Source: CAD feature listing. Evaluate the final solid. Frame: model axes, mm. A direction names the side the tool comes from. Coordinates: 2 decimals unless noted, no trailing zeros. Write each loop counter-clockwise with the first axis right and the second up, starting at its lowest first coordinate (ties: lowest second). Pieces come first, ordered by that corner, then holes. Notation, with made-up numbers: M 84.5,57.25 L 107.5,57.25 A24 cw 107.5,94.25 Z; hole C -16.5,-10.5 d6. An arc over 180 degrees is marked long. Answer as CSV lines item,"result". Start each with the question number.
1. Section C-C on z = 0.6. Return the cut outline in (x, y), plus the area to 3 significant figures.
2. Section A-A on x = 7.5. Return the cut outline in (y, z), plus the area to 3 significant figures.
3. Section B-B on y = 32. Return the cut outline in (x, z).
4. Reachability of faces 1 (the face through (59, -3, 1)), 2 (the face through (1, 70, 1)) from +Z, -Z, +X, -X, +Y, -Y: full face, straight path, thin tool, end or side. Return the list, or none.
5. Line query: probe 1 along X at (y, z) = (62, 1.15); probe 2 along Y at (x, z) = (-52, 1.1); probe 3 along Y at (x, z) = (-3.5, 2.4). Output: solid intervals per line, ascending. Write a range as [from, to].
6. Mould query, pull axis X, two halves, no side actions, for faces 3 (the face through (-10, 66, 1)), 4 (the face through (-64, -73, 1)), 5 (the face through (-60, -3, 1)), 6 (the face through (-1, -75, 1)). Classes: pulls with the +X half, pulls with the -X half, needs draft (parallel to the pull), parting line crosses it, or undercut.
```python
from build123d import *

# Parameters (mm, degrees)
SKETCH1_R           = 1.5
SKETCH1_W           = 20
SKETCH1_H           = 3.2
SKETCH1_W_2         = 3.2
SKETCH1_H_2         = 70
BOSS_EXTRUDE1_DEPTH = 3


with BuildPart() as part:
    # Sketch1 → Boss-Extrude1 (new body)
    with BuildSketch(Plane.XY):
        with BuildLine():
            Line((-60, -75), (60, -75))
            ThreePointArc((60, -75), (63.535533906, -73.535533906), (65, -70))
            Line((65, -70), (65, 70))
            Line((65, 70), (-65, 70))
            Line((-65, 70), (-65, -70))
            ThreePointArc((-65, -70), (-63.535533906, -73.535533906), (-60, -75))
        make_face()
        with Locations((-52, -31)):
            Circle(SKETCH1_R, mode=Mode.SUBTRACT)
        with Locations((52, -31)):
            Circle(SKETCH1_R, mode=Mode.SUBTRACT)
        with Locations((52, 60)):
            Circle(SKETCH1_R, mode=Mode.SUBTRACT)
        with Locations((-52, 60)):
            Circle(SKETCH1_R, mode=Mode.SUBTRACT)
        with Locations((0, 66.4)):
            Rectangle(SKETCH1_W, SKETCH1_H, mode=Mode.SUBTRACT)
        with Locations((-59.5, 32)):
            Rectangle(SKETCH1_W_2, SKETCH1_H_2, mode=Mode.SUBTRACT)
        with Locations((59.5, 32)):
            Rectangle(SKETCH1_W_2, SKETCH1_H_2, mode=Mode.SUBTRACT)
    extrude(amount=BOSS_EXTRUDE1_DEPTH)


solid = part.part
```
Values:
1,outline,"M -65,-70 A5 ccw -60,-75 L 60,-75 A5 ccw 65,-70 L 65,70 L -65,70 Z; hole M -61.1,-3 L -57.9,-3 L -57.9,67 L -61.1,67 Z; hole C -52,-31 d3; hole C -52,60 d3; hole M -10,64.8 L 10,64.8 L 10,68 L -10,68 Z; hole C 52,-31 d3; hole C 52,60 d3; hole M 57.9,-3 L 61.1,-3 L 61.1,67 L 57.9,67 Z"
1,area,"18,300 mm²"
2,outline,"M -75,0 L 64.8,0 L 64.8,3 L -75,3 Z; M 68,0 L 70,0 L 70,3 L 68,3 Z"
2,area,"425 mm²"
3,outline,"M -65,0 L -61.1,0 L -61.1,3 L -65,3 Z; M -57.9,0 L 57.9,0 L 57.9,3 L -57.9,3 Z; M 61.1,0 L 65,0 L 65,3 L 61.1,3 Z"
4,face 1,"+Z, -Z"
4,face 2,"+Z, -Z, +X, -X, +Y"
5,probe 1,"[-65, -61.1], [-57.9, 57.9], [61.1, 65]"
5,probe 2,"[-75, -32.5], [-29.5, 58.5], [61.5, 70]"
5,probe 3,"[-75, 64.8], [68, 70]"
6,face 3,"undercut"
6,face 4,"pulls with the -X half"
6,face 5,"undercut"
6,face 6,"needs draft"
